Here's how the part is built. I have some questions about the finished solid (model axes, mm). Round coordinates to 2 decimals unless told otherwise and drop trailing zeros. Write each loop counter-clockwise with the first axis right and the second up, starting at its lowest first coordinate (ties: lowest second). Pieces come first, ordered by that corner, then holes. Notation, with made-up numbers: M 47,-40 L 101,-40 A25 ccw 101,-14 Z; hole C -24,33.25 d1. An arc over 180 degrees is marked long. Use a Markdown table: item, result. Add a question column.
```python
from build123d import *

# Parameters (mm, degrees)
SKETCH1_R           = 3.175
BOSS_EXTRUDE1_DEPTH = 6
SERVO_MOUNT_REACH   = 203.398
SKETCH2_R           = 0.5
LPATTERN1_COUNT     = 6
LPATTERN1_PITCH     = 22


with BuildPart() as part:
    # Sketch1 → Boss-Extrude1 (new body)
    with BuildSketch(Plane(origin=(0, 0, 0), x_dir=(0, 0, -1), z_dir=(1, 0, 0))):
        with BuildLine():
            Line((-3.175, 0), (-20, 0))
            Line((-20, 0), (-20, 48))
            ThreePointArc((-20, 48), (-19.414213562, 49.414213562), (-18, 50))
            Line((-18, 50), (193, 50))
            ThreePointArc((193, 50), (194.414213562, 49.414213562), (195, 48))
            Line((195, 48), (195, 0))
            Line((195, 0), (178.175, 0))
            Line((178.175, 0), (178.175, 10))
            Line((178.175, 10), (179.9, 10))
            ThreePointArc((179.9, 10), (184.9, 15), (179.9, 20))
            Line((179.9, 20), (170.1, 20))
            ThreePointArc((170.1, 20), (165.1, 15), (170.1, 10))
            Line((170.1, 10), (171.825, 10))
            Line((171.825, 10), (171.825, 0))
            Line((171.825, 0), (3.175, 0))
            Line((3.175, 0), (3.175, 10))
            Line((3.175, 10), (4.9, 10))
            ThreePointArc((4.9, 10), (9.9, 15), (4.9, 20))
            Line((4.9, 20), (-4.9, 20))
            ThreePointArc((-4.9, 20), (-9.9, 15), (-4.9, 10))
            Line((-4.9, 10), (-3.175, 10))
            Line((-3.175, 10), (-3.175, 0))
        make_face()
        with Locations(Location((175, 30, 0), (0, 0, 180))):
            Circle(SKETCH1_R, mode=Mode.SUBTRACT)
        with Locations((0, 30)):
            Circle(SKETCH1_R, mode=Mode.SUBTRACT)
    extrude(amount=BOSS_EXTRUDE1_DEPTH)

    # Sketch2 → servo mount (cut, up to next)
    with BuildSketch(Plane(origin=(6, 0, 0), x_dir=(0, 0, -1), z_dir=(1, 0, 0)), mode=Mode.PRIVATE) as servo_mount_sk1:
        with Locations((30, 38.9)):
            Circle(SKETCH2_R)
    servo_mount_tool1 = extrude(servo_mount_sk1.sketch, amount=-SERVO_MOUNT_REACH, mode=Mode.PRIVATE) & part.part
    # Sketch2 → servo mount (cut, up to next)
    with BuildSketch(Plane(origin=(6, 0, 0), x_dir=(0, 0, -1), z_dir=(1, 0, 0)), mode=Mode.PRIVATE) as servo_mount_sk2:
        with Locations((30, 11.1)):
            Circle(SKETCH2_R)
    servo_mount_tool2 = extrude(servo_mount_sk2.sketch, amount=-SERVO_MOUNT_REACH, mode=Mode.PRIVATE) & part.part
    # Sketch2 → servo mount (cut, up to next)
    with BuildSketch(Plane(origin=(6, 0, 0), x_dir=(0, 0, -1), z_dir=(1, 0, 0)), mode=Mode.PRIVATE) as servo_mount_sk3:
        with BuildLine():
            Line((24, 13), (36, 13))
            ThreePointArc((36, 13), (36.353553391, 13.146446609), (36.5, 13.5))
            Line((36.5, 13.5), (36.5, 36.5))
            ThreePointArc((36.5, 36.5), (36.353553391, 36.853553391), (36, 37))
            Line((36, 37), (24, 37))
            ThreePointArc((24, 37), (23.646446609, 36.853553391), (23.5, 36.5))
            Line((23.5, 36.5), (23.5, 13.5))
            ThreePointArc((23.5, 13.5), (23.646446609, 13.146446609), (24, 13))
        make_face()
    servo_mount_tool3 = extrude(servo_mount_sk3.sketch, amount=-SERVO_MOUNT_REACH, mode=Mode.PRIVATE) & part.part
    servo_mount_1 = servo_mount_tool1.solids().sort_by_distance((6, 38.9, -30))[0]
    add(servo_mount_1, mode=Mode.SUBTRACT)
    servo_mount_2 = servo_mount_tool2.solids().sort_by_distance((6, 11.1, -30))[0]
    add(servo_mount_2, mode=Mode.SUBTRACT)
    servo_mount_3 = servo_mount_tool3.solids().sort_by_distance((6, 25, -30))[0]
    add(servo_mount_3, mode=Mode.SUBTRACT)
    servo_mount = servo_mount_1 + servo_mount_2 + servo_mount_3  # servo mount as one shape, for the pattern or mirror that repeats it

    # LPattern1: servo mount ×6
    with Locations(*[(0, 0, -i * LPATTERN1_PITCH) for i in range(1, LPATTERN1_COUNT)]):
        add(servo_mount, mode=Mode.SUBTRACT)


solid = part.part
```
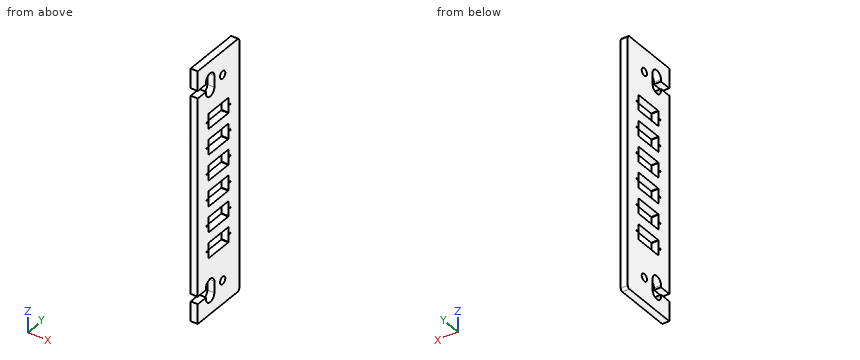
Item 1: Imagine slicing it at A-A on z = -49. List the corners of the cut face in (x, y) for me.
Item 2: Imagine slicing it at D-D on x = 3.7. Count the separate pieces of the cut face and the enclosed holes in it, plus the area to 3 significant figures.
Item 3: For pin 1 Ø2 at (x, z) = (2, -2.5) entering from -Y, with a flat end and sliding along its axis, tell me the tip position at first contact or that it passes through.
Item 4: I need wall thicknesses on probe 1 along Y at (x, z) = (4.75, -96); probe 2 along Z at (x, y) = (1.55, 3) (3 decimals); probe 3 along Y at (x, z) = (1.55, -5). Which ranges of each line are inside material? Lowest first, please. Write a range as from..to.
Item 5: Imagine slicing it at B-B on y = 22. List the corners of the cut face in (x, z) for me.
Item 6: Imagine slicing it at C-C on z = -175. List the corners of the cut face in (x, y) for me (3 decimals).
The answers:
| question | item | result |
|---|---|---|
| 1 | outline | M 0,0 L 6,0 L 6,13 L 0,13 Z; M 0,37 L 6,37 L 6,50 L 0,50 Z |
| 2 | separate pieces | 1 |
| 2 | enclosed holes | 20 |
| 2 | area | 8,320 mm² |
| 3 | pin 1 | y = 0 |
| 4 | probe 1 | 0..10.6, 11.6..13, 37..38.4, 39.4..50 |
| 4 | probe 2 | -195..-178.175, -171.825..-3.175, 3.175..20 |
| 4 | probe 3 | 0..10, 20..50 |
| 5 | outline | M 0,-195 L 6,-195 L 6,-146.5 L 0,-146.5 Z; M 0,-133.5 L 6,-133.5 L 6,-124.5 L 0,-124.5 Z; M 0,-111.5 L 6,-111.5 L 6,-102.5 L 0,-102.5 Z; M 0,-89.5 L 6,-89.5 L 6,-80.5 L 0,-80.5 Z; M 0,-67.5 L 6,-67.5 L 6,-58.5 L 0,-58.5 Z; M 0,-45.5 L 6,-45.5 L 6,-36.5 L 0,-36.5 Z; M 0,-23.5 L 6,-23.5 L 6,20 L 0,20 Z |
| 6 | outline | M 0,20 L 6,20 L 6,26.825 L 0,26.825 Z; M 0,33.175 L 6,33.175 L 6,50 L 0,50 Z |
